Verification items for this drawing (mm, ordinates from the low corner). Coordinates: 2 decimals unless noted, no trailing zeros. Loops run counter-clockwise (first coordinate to the right, second up) from the corner with the lowest first, then second, coordinate; pieces in that order, holes last. Notation, with made-up numbers: M -19.75,44.25 L 4.25,44.25 A21 cw 4.25,54.25 Z; hole C 50.5,-36.5 d11. An arc over 180 degrees is marked long. One line per question, with ' | ' between items. Start each with the question number.
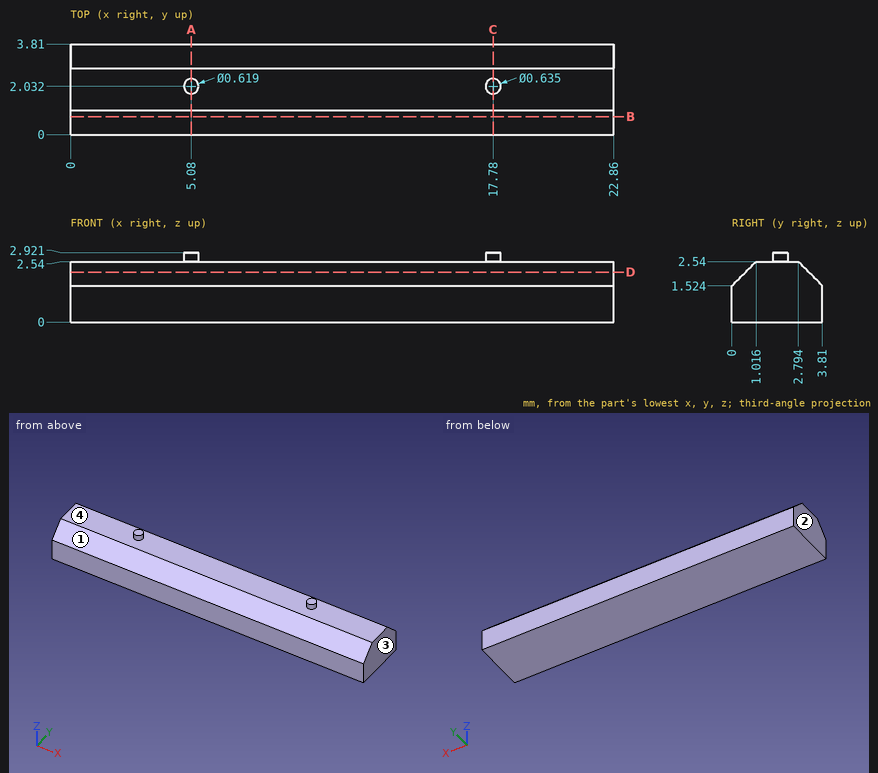
1. Sectioned sample at B-B (y = 0.75). Record the cut outline in (x, z).
2. Thickness scan on line 1 (Z direction, x = 21.5, y = 1.9); line 2 (Z direction, x = 7.5, y = 0.75) (1 decimal); line 3 (Y direction, x = 5.75, z = 2.15) (1 decimal). Record the ranges inside material, lowest first.
3. Depth check by flat-ended pin: pin 1 Ø0.9 at (x, y) = (9, 2) entering from +Z; pin 2 Ø1.5 at (x, z) = (8.5, 2.5) entering from -Y; pin 3 Ø1 at (y, z) = (3.5, 0.5) entering from -X. Enter the tip coordinate at first touch or a pass-through.
4. Sectioned sample at D-D (z = 2.1). Record the cut outline in (x, y).
5. Sectioned sample at C-C (x = 17.78). Record the cut outline in (y, z).
6. Draft check along X on the marked faces 1, 2, 3 and 4. Enter one of: +X half, -X half, draft (parallel to the pull), parting line (faces both ways), or undercut.
7. Sectioned sample at A-A (x = 5.08). Record the cut outline in (y, z).
Result:
1) outline: M 0,0 L 22.86,0 L 22.86,2.27 L 0,2.27 Z
2) line 1: z = 0 to 2.54 | line 2: z = 0 to 2.3 | line 3: y = 0.6 to 3.2
3) pin 1: stops at z = 2.54 | pin 2: stops at y = 0.23 | pin 3: stops at x = 0
4) outline: M 0,0.58 L 22.86,0.58 L 22.86,3.23 L 0,3.23 Z
5) outline: M 0,0 L 3.81,0 L 3.81,1.52 L 2.79,2.54 L 2.35,2.54 L 2.35,2.92 L 1.71,2.92 L 1.71,2.54 L 1.02,2.54 L 0,1.52 Z
6) face 1: draft | face 2: -X half | face 3: +X half | face 4: undercut
7) outline: M 0,0 L 3.81,0 L 3.81,1.52 L 2.79,2.54 L 2.34,2.54 L 2.34,2.92 L 1.72,2.92 L 1.72,2.54 L 1.02,2.54 L 0,1.52 Z
